For this review, take the finished solid that the model builds, in its own axes (mm). Round coordinates to 2 decimals unless told otherwise and drop trailing zeros. Order: outer loops, then holes, each group sorted by start corner. A loop starts at its lowest first (then second) coordinate and runs counter-clockwise, first axis right, second up. Notation, with made-up numbers: (87.25, -11) -> (97.25, -11) arc R23 ccw to (97.25, 17) -> close; hole circle Ø11 at (-10.5, 8.25). An arc over 180 degrees is marked (long way). Use a Markdown table: item, result. Add a question column.
1) Wall thickness on line 1 along Z through (x, y) = (126, -2.5); line 2 along X through (y, z) = (-2.1, -110.5); line 3 along X through (y, z) = (-2.1, -95.5): over which ranges is each line inside the solid? List them lowest first. Write a range as [from, to].
2) Clearance check with flat-ended pins moving along their axes: P1, Ø1, axis at x = 88, y = -1.5, coming from the -Z side; P2, Ø1.6, axis at y = -1.5, z = -115, coming from the +X side; P3, Ø1.6, axis at y = -1, z = -124.5, coming from the -X side. State where each tip first meets the part, or that it passes through.
3) Consider section B-B (x = 281). State the section outline as (y, z) points (3 decimals), plus the area to 4 significant figures.
4) Consider section A-A (y = -2.5). State the section outline as (x, z) points.
```python
from build123d import *

# Parameters (mm, degrees)
BASE_FLANGE1_DEPTH = 3.175
FILLET1_R          = 5


# Sheet-metal steps are written as plain solids
with BuildPart() as part:
    # Sketch1 → Base-Flange1 (new body)
    with BuildSketch(Plane(origin=(0, 0, 0), x_dir=(1, 0, 0), z_dir=(0, 1, 0))):
        Polygon((215, 100), (350, 100), (350, 0), (0, 0), (0, 100), (135, 100), (135, 150), (215, 150), align=None)
    extrude(amount=-BASE_FLANGE1_DEPTH)

    # Fillet1
    fillet1_edges = [part.edges().sort_by_distance(p)[0] for p in [
        (0, -1.5875, -100),
        (135, -1.5875, -150),
        (215, -1.5875, -150),
        (350, -1.5875, -100),
        (350, -1.5875, 0),
        (0, -1.5875, 0),
    ]]
    fillet(fillet1_edges, radius=FILLET1_R)


solid = part.part
```
Results list:
| question | item | result |
|---|---|---|
| 1 | line 1 | [-100, 0] |
| 1 | line 2 | [135, 215] |
| 1 | line 3 | [0.03, 349.97] |
| 2 | P1 | z = -100 |
| 2 | P2 | x = 215 |
| 2 | P3 | x = 135 |
| 3 | outline | (-3.175, -100) -> (0, -100) -> (0, 0) -> (-3.175, 0) -> close |
| 3 | area | 317.5 mm2 |
| 4 | outline | (0, -95) arc R5 ccw to (5, -100) -> (135, -100) -> (135, -145) arc R5 ccw to (140, -150) -> (210, -150) arc R5 ccw to (215, -145) -> (215, -100) -> (345, -100) arc R5 ccw to (350, -95) -> (350, -5) arc R5 ccw to (345, 0) -> (5, 0) arc R5 ccw to (0, -5) -> close |
